The figure shows three views and two pictorial views of one solid part (mm, origin at its lowest corner). Answer the questions. A direction names the side the tool comes from. Round coordinates to 2 decimals unless told otherwise and drop trailing zeros. Order: outer loops, then holes, each group sorted by start corner. A loop starts at its lowest first (then second) coordinate and runs counter-clockwise, first axis right, second up. Notation, with made-up numbers: (-12.5, 5.25) -> (18.5, 5.25) arc R8 ccw to (18.5, 14.25) -> close; hole circle Ø5 at (52, 4). An arc over 180 degrees is marked (long way). One line per item, written item: value. Start each with the question number.
1. Section D-D (z = 16) is taken. Give the vertices of the cut face in (x, y).
2. Flat-ended cylindrical pins translate along their axes: pin 1 Ø8 at (x, z) = (38, 18.5) entering from +Y; pin 2 Ø3.5 at (x, y) = (30, 50) entering from -Z; pin 3 Ø3 at (y, z) = (48.5, 1.5) entering from -X; pin 4 Ø10 at (y, z) = (8, 12.5) entering from +X. Find the tip coordinate at first contact, or state that the pin passes through.
3. Section C-C (y = 30) is taken. Give the vertices of the cut face in (x, z), then the cut area to 3 significant figures.
4. Consider line 1 (Y direction, x = 10, z = 2.5); line 2 (Z direction, x = 37, y = 10); line 3 (Y direction, x = 46.5, z = 4.25). Determine where each line is inside the solid, lowest interval first.
5. Section B-B (x = 50) is taken. Give the vertices of the cut face in (y, z), then the cut area to 3 significant figures.
6. Section A-A (y = 50) is taken. Give the vertices of the cut face in (x, z).
7. The mould has two halves that part along X. Classify the marked faces 4, 5 and 6: released by +X, released by -X, zero draft, split by the parting line, or undercut.
8. For the marked faces 1, 2 and 3, determine the directions among +Z, -Z, +X, -X, +Y, -Y from which every point of the face is accessible in a straight line to the end or side of a thin tool.
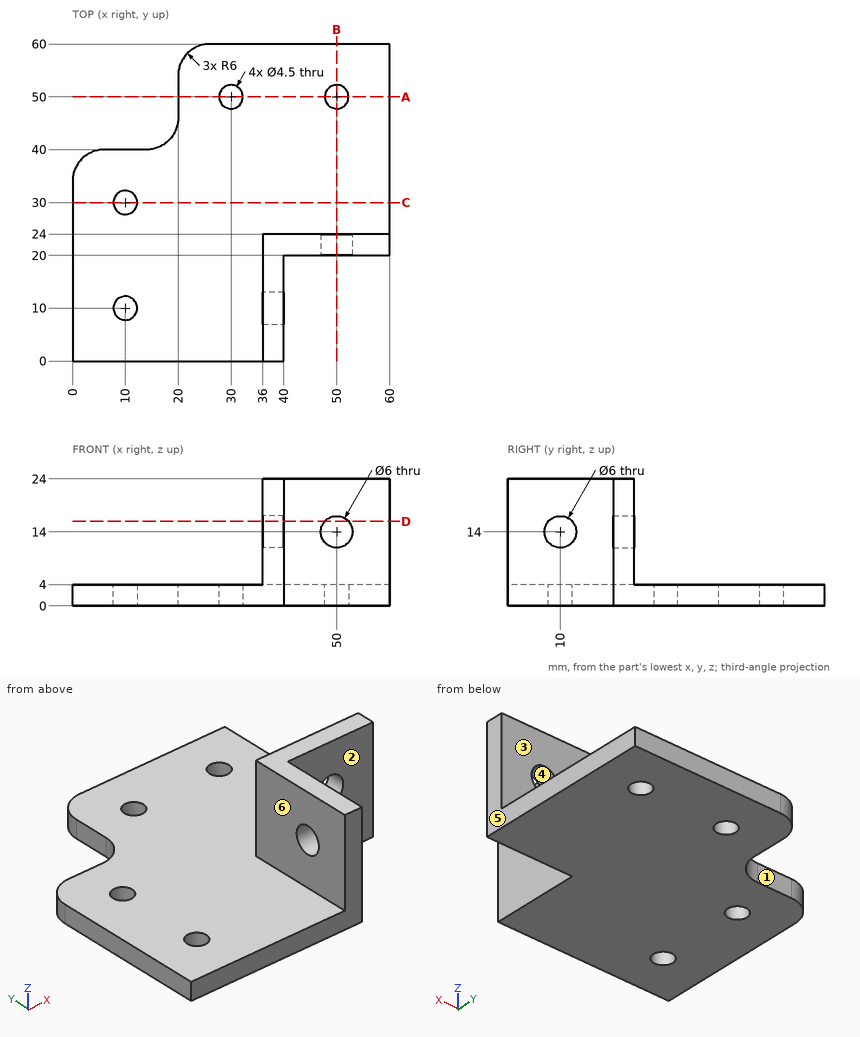
Answer:
1. outline: (36, 0) -> (40, 0) -> (40, 7.76) -> (36, 7.76) -> close; (36, 12.24) -> (40, 12.24) -> (40, 20) -> (47.76, 20) -> (47.76, 24) -> (36, 24) -> close; (52.24, 20) -> (60, 20) -> (60, 24) -> (52.24, 24) -> close
2. pin 1: y = 24
2. pin 2: through
2. pin 3: x = 20
2. pin 4: x = 40
3. outline: (0, 0) -> (7.75, 0) -> (7.75, 4) -> (0, 4) -> close; (12.25, 0) -> (60, 0) -> (60, 4) -> (12.25, 4) -> close
3. area: 222 mm^2
4. line 1: 0 to 7.75, 12.25 to 27.75, 32.25 to 40
4. line 2: 0 to 11, 17 to 24
4. line 3: 20 to 24
5. outline: (20, 0) -> (47.75, 0) -> (47.75, 4) -> (24, 4) -> (24, 11) -> (20, 11) -> close; (20, 17) -> (24, 17) -> (24, 24) -> (20, 24) -> close; (52.25, 0) -> (60, 0) -> (60, 4) -> (52.25, 4) -> close
5. area: 198 mm^2
6. outline: (20, 0) -> (27.75, 0) -> (27.75, 4) -> (20, 4) -> close; (32.25, 0) -> (47.75, 0) -> (47.75, 4) -> (32.25, 4) -> close; (52.25, 0) -> (60, 0) -> (60, 4) -> (52.25, 4) -> close
7. face 4: undercut
7. face 5: released by +X
7. face 6: released by -X
8. face 1: +Z, -Z, -X, +Y
8. face 2: +Z, -Z, +X, -Y
8. face 3: +Z, +X, -X, +Y
